CAD build for the part. Positions are in the model's coordinates, mm. A direction names the side the tool comes from. Round coordinates to 2 decimals unless told otherwise and drop trailing zeros. Write each loop counter-clockwise with the first axis right and the second up, starting at its lowest first coordinate (ties: lowest second). Pieces come first, ordered by that corner, then holes. Notation, with made-up numbers: M -27.75,14 L 12.25,14 A6 cw 12.25,18 Z; hole C 0.25,79.5 d8. An arc over 180 degrees is marked long. Write each question's results on one line, items separated by ' | '. Start each with the question number.
```python
from build123d import *

# Parameters (mm, degrees)
SKETCH1_W           = 20
SKETCH1_H           = 9.6
SKETCH1_R           = 1.15
BOSS_EXTRUDE1_DEPTH = 3
FILLET1_R           = 2
SKETCH2_R           = 1.9
CUT_EXTRUDE1_DEPTH  = 1


with BuildPart() as part:
    # Sketch1 → Boss-Extrude1 (new body)
    with BuildSketch(Plane.XY):
        with Locations((10, 4.8)):
            Rectangle(SKETCH1_W, SKETCH1_H)
        with Locations((6.85, 4.8)):
            Circle(SKETCH1_R, mode=Mode.SUBTRACT)
        with Locations((13.15, 4.8)):
            Circle(SKETCH1_R, mode=Mode.SUBTRACT)
    extrude(amount=BOSS_EXTRUDE1_DEPTH)

    # Fillet1
    fillet1_edges = [part.edges().sort_by_distance(p)[0] for p in [
        (20, 0, 1.5),
        (0, 0, 1.5),
    ]]
    fillet(fillet1_edges, radius=FILLET1_R)

    # Sketch2 → Cut-Extrude1 (cut)
    with BuildSketch(Plane.XY.offset(3)):
        with Locations((6.85, 4.8)):
            Circle(SKETCH2_R)
        with Locations((13.15, 4.8)):
            Circle(SKETCH2_R)
    extrude(amount=-CUT_EXTRUDE1_DEPTH, mode=Mode.SUBTRACT)


solid = part.part
```
1) Pull direction X, two halves, no side cores. Call faces 1 (the face through (10, 5, 0)), 2 (the face through (7.912, 4.36, 0.986)), 3 (the face through (0.57, 0.6, 1.52)), 4 (the face through (12.24, 4.1, 0.99)): pulls with the +X half, pulls with the -X half, needs draft (parallel to the pull), parting line crosses it, or undercut.
2) Saw through at C-C, the plane y = 4. Write the cut outline in (x, z), plus the area to 3 significant figures.
3) Wall check: line 1 along Y through (x, z) = (6.85, 2.45); line 2 along Y through (x, z) = (6.85, 0.85); line 3 along X through (y, z) = (4.8, 1.1). Give the ranges that are in metal, low to high. Write a range as from..to.
4) Drop flat-ended pins along their axis: pin 1 Ø1.1 at (x, y) = (7, 5) entering from +Z; pin 2 Ø3.5 at (x, y) = (13.15, 4.8) entering from +Z. Give the stop position or say it passes through.
5) 3-axis set-ups, long thin cutter, end or side, ignore diameter. For faces 5 (the face through (20, 6, 1)), 6 (the face through (14, 6, 2)): which of +Z, -Z, +X, -X, +Y, -Y reach the whole face in a straight line?
6) Saw through at D-D, the plane x = 14.5. Write the cut outline in (y, z), plus the area to 3 significant figures.
7) Saw through at B-B, the plane z = 0.8. Write the cut outline in (x, y).
8) Saw through at A-A, the plane x = 6.85. Write the cut outline in (y, z), plus the area to 3 significant figures.
Filled sheet:
1) face 1: needs draft | face 2: undercut | face 3: pulls with the -X half | face 4: undercut
2) outline: M 0,0 L 6.02,0 L 6.02,2 L 5.13,2 L 5.13,3 L 0,3 Z; M 7.68,0 L 12.32,0 L 12.32,2 L 11.43,2 L 11.43,3 L 8.57,3 L 8.57,2 L 7.68,2 Z; M 13.98,0 L 20,0 L 20,3 L 14.87,3 L 14.87,2 L 13.98,2 Z | area: 46.5 mm^2
3) line 1: y = 0..2.9, 6.7..9.6 | line 2: y = 0..3.65, 5.95..9.6 | line 3: x = 0..5.7, 8..12, 14.3..20
4) pin 1: passes through | pin 2: stops at z = 2
5) face 5: +Z, -Z, +X, +Y, -Y | face 6: +Z
6) outline: M 0,0 L 9.6,0 L 9.6,3 L 6.14,3 L 6.14,2 L 3.46,2 L 3.46,3 L 0,3 Z | area: 26.1 mm^2
7) outline: M 0,2 A2 ccw 2,0 L 18,0 A2 ccw 20,2 L 20,9.6 L 0,9.6 Z; hole C 6.85,4.8 d2.3; hole C 13.15,4.8 d2.3
8) outline: M 0,0 L 3.65,0 L 3.65,2 L 2.9,2 L 2.9,3 L 0,3 Z; M 5.95,0 L 9.6,0 L 9.6,3 L 6.7,3 L 6.7,2 L 5.95,2 Z | area: 20.4 mm^2
